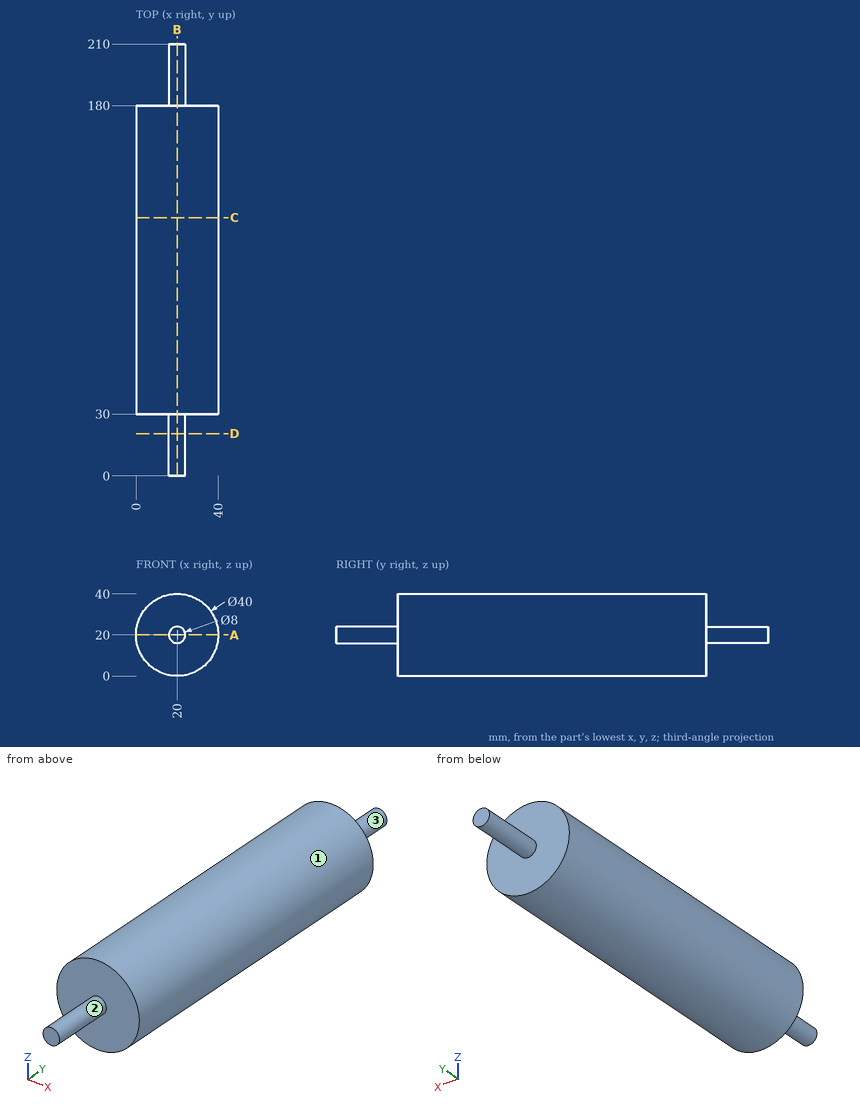
Geometry: see drawing. Coordinates: mm, zero at the bounding-box minimum. A direction names the side the tool comes from. Give positions to 0.01 mm unless a question says otherwise; leave off trailing zeros. Write each loop counter-clockwise with the first axis right and the second up, starting at its lowest first coordinate (ties: lowest second). Pieces come first, ordered by that corner, then holes. Notation, with made-up numbers: M 68,32 L 81,32 A30 cw 81,59 Z; hole C 2,-26.5 d9. An arc over 180 degrees is marked long. Return JSON: item names as keys, results as strings. Group by question number.
1) Set-up query: the marked faces 1, 2 and 3. Return all of +Z, -Z, +X, -X, +Y, -Y with unobstructed straight access to the full face (end or side cutting, diameter ignored); none if empty.
2) Cut plane D-D, the plane y = 20.5. Output: boundary loops of the cut face in (x, z).
3) First-contact query: pin 1 Ø1 at (x, y) = (32.5, 62.5) entering from +Z; pin 2 Ø4 at (y, z) = (23.5, 18.5) entering from -X; pin 3 Ø10 at (x, y) = (27, 123.5) entering from +Z. Flat tips, straight axial feed; report the tip coordinate or a pass-through.
4) Cut plane A-A, the plane z = 20. Output: boundary loops of the cut face in (x, y), then the cut area to 3 significant figures.
5) Cut plane C-C, the plane y = 125.5. Output: boundary loops of the cut face in (x, z), then the cut area to 3 significant figures.
6) Ray query, L1, parallel to Y at x = 18.5, z = 25.5; L2, parallel to Z at x = 23, y = 88; L3, parallel to Z at x = 37, y = 85. Return the intervals inside material, ascending.
7) Cut plane B-B, the plane x = 20. Output: boundary loops of the cut face in (y, z).
Data:
{
 "1": {"face 1": "+Y, -Y", "face 2": "-Y", "face 3": "+Y"},
 "2": {"outline": "C 20,20 d8"},
 "3": {"pin 1": "stops at z = 36", "pin 2": "stops at x = 16", "pin 3": "stops at z = 39.9"},
 "4": {"outline": "M 0,30 L 16,30 L 16,0 L 24,0 L 24,30 L 40,30 L 40,180 L 24,180 L 24,210 L 16,210 L 16,180 L 0,180 Z", "area": "6,480 mm²"},
 "5": {"outline": "C 20,20 d40", "area": "1,260 mm²"},
 "6": {"L1": "y = 30 to 180", "L2": "z = 0.23 to 39.77", "L3": "z = 9.46 to 30.54"},
 "7": {"outline": "M 0,16 L 30,16 L 30,0 L 180,0 L 180,16 L 210,16 L 210,24 L 180,24 L 180,40 L 30,40 L 30,24 L 0,24 Z"}
}
